For this review, take the finished solid that the model builds, in its own axes (mm). A direction names the side the tool comes from. Round coordinates to 2 decimals unless told otherwise and drop trailing zeros. Write each loop counter-clockwise with the first axis right and the second up, starting at its lowest first coordinate (ties: lowest second). Pieces come first, ordered by that corner, then holes. Notation, with made-up numbers: M -10.75,30 L 15.25,30 A27 cw 15.25,54 Z; hole C 75.5,78 d9. An arc over 180 degrees is marked long. One line per question, with ' | ' between items.
Autodesk Fusion 360 part; units mm, degrees
sketch "Sketch1" plane through (0, 0, 0) normal (0, 0, 1) x (1, 0, 0)
  line L0 (20, 20) -> (-20, 20)
  line L1 (-20, 20) -> (-20, -20)
  line L2 (-20, -20) -> (20, -20)
  line L3 (20, -20) -> (20, 20)
  line L4 (20, 20) -> (-20, -20) construction
  line L5 (-20, 20) -> (20, -20) construction
  circle A0 centre (0, 0) radius 4
  circle A1 centre (0, 0) radius 9.4
  line L6 (13, -13) -> (-13, -13) construction
  line L7 (-13, -13) -> (-13, 13) construction
  line L8 (-13, 13) -> (13, 13) construction
  line L9 (13, 13) -> (13, -13) construction
  line L10 (13, -13) -> (-13, 13) construction
  line L11 (-13, -13) -> (13, 13) construction
  circle A2 centre (-13, 13) radius 1
  circle A3 centre (13, 13) radius 1
  circle A4 centre (13, -13) radius 1
  circle A5 centre (-13, -13) radius 1
  dimension "d1" = 40
  dimension "d2" = 40
  dimension "d3" = 8
  dimension "d4" = 18.8
  dimension "d9" = 26
  dimension "d10" = 26
  dimension "d11" = 2
  dimension "d12" = 2
  dimension "d13" = 2
  dimension "d14" = 2
extrude "Extrude1" add sketch "Sketch1" along normal blind 9 contours A1
extrude "Extrude2" add sketch "Sketch1" along normal blind 18 contours L0 L1 L2 L3
equation "d12 = d11"
equation "d13 = d11"
equation "d14 = d11"
Item 1: Take a section at B-B (z = 4). Write out the cut boundary in (x, y).
Results:
outline: M -20,-20 L 20,-20 L 20,20 L -20,20 Z; hole C -13,-13 d2; hole C -13,13 d2; hole C 0,0 d8; hole C 13,-13 d2; hole C 13,13 d2
Item 2: Mouldability with a two-part tool opening along X and no side actions: class faces 3 (the face through (-2.038, 9.176, 13.437)), 4 (the face through (-5, 9, 18)), 5 (the face through (20, 0, 9)) as +X half, -X half, draft (parallel to the pull), parting line (faces both ways), or undercut.
Results:
face 3: undercut | face 4: draft | face 5: +X half
Item 3: Take a section at A-A (y = 0). Write out the cut boundary in (x, z), then the cut area to 3 significant figures.
Results:
outline: M -20,0 L -4,0 L -4,9 L -9.4,9 L -9.4,18 L -20,18 Z; M 4,0 L 20,0 L 20,18 L 9.4,18 L 9.4,9 L 4,9 Z | area: 479 mm2
Item 4: Take a section at D-D (y = -13). Write out the cut boundary in (x, z).
Results:
outline: M -20,0 L -14,0 L -14,18 L -20,18 Z; M -12,0 L 12,0 L 12,18 L -12,18 Z; M 14,0 L 20,0 L 20,18 L 14,18 Z
Item 5: Machinability: for faces 1 (the face through (-20, 0, 9)), 2 (the face through (2, -4, 9)), which of the approach directions +Z, -Z, +X, -X, +Y, -Y give a long, thin tool a straight path to every point of the face, cutting with its end or side? Answer none if there is none.
Results:
face 1: +Z, -Z, -X, +Y, -Y | face 2: +Z
Item 6: To check wall thickness, follow line 1 along Y through (x, z) = (-13, 4); line 2 along Y through (x, z) = (0, 3); line 3 along Z through (x, y) = (7, 3). State the ranges of each line that lie inside material, in increasing order. Write a range as from..to.
Results:
line 1: -20..-14, -12..12, 14..20 | line 2: -20..-4, 4..20 | line 3: 0..9
Item 7: Insertion check: pin 1 Ø5.5 at (x, y) = (2, -0.5) entering from +Z. The pin has a flat end and moves straight along its axis. Give the tip position at first contact, or say it passes through.
Results:
pin 1: z = 9
